```python
from build123d import *

# Parameters (mm, degrees)
F0_R     = 0.8
F1_DEPTH = 13
F2_R     = 0.8
F3_DEPTH = 6.5
F4_R     = 1.13
F5_DEPTH = 0.4


with BuildPart() as f1:
    # F0 (on Right) → F1 (new body)
    with BuildSketch(Plane.YZ):
        with BuildLine():
            ThreePointArc((0, 2.4), (-1.2, 1.2), (0, 0))
            Line((0, 0), (6.1, 0))
            Line((6.1, 0), (6.1, 0.4))
            Line((6.1, 0.4), (0.894427, 0.4))
            ThreePointArc((0.894427, 0.4), (1.095445, 1.689898), (0, 2.4))
        make_face()
        with Locations((0, 1.2)):
            Circle(F0_R, mode=Mode.SUBTRACT)
    extrude(amount=F1_DEPTH)

    # F2 (on face) → F3 (cut)
    with BuildSketch(Plane.YZ.offset(13)):
        with BuildLine():
            Line((0.894427, 0), (0.894427, 0.4))
            ThreePointArc((0.894427, 0.4), (-0.489898, 2.295445), (0, 0))
            Line((0, 0), (0.894427, 0))
        make_face()
        with Locations((0, 1.2)):
            Circle(F2_R, mode=Mode.SUBTRACT)
    extrude(amount=-F3_DEPTH, mode=Mode.SUBTRACT)

    # F4 (on face) → F5 (cut, through all)
    with BuildSketch(Plane.XY.offset(0.4)):
        with Locations((2.375, 3.67)):
            Circle(F4_R)
        with Locations((10.625, 3.67)):
            Circle(F4_R)
    extrude(amount=-F5_DEPTH, mode=Mode.SUBTRACT)


solid = f1.part
```
Geometry: final body of the model. Coordinates: model frame, mm. A direction names the side the tool comes from. Coordinates: 2 decimals unless noted, no trailing zeros. Write each loop counter-clockwise with the first axis right and the second up, starting at its lowest first coordinate (ties: lowest second). Pieces come first, ordered by that corner, then holes. Notation, with made-up numbers: M -34.5,25.25 L 1.5,25.25 A13 ccw 1.5,29.25 Z; hole C -27.5,25 d11. An arc over 180 degrees is marked long. Use CSV: the item, a comma, the result in double quotes. Start each with the question number.
1. Reachability of faces 1 (the face through (6, 3, 0)), 2 (the face through (6.5, 1, 1)) from +Z, -Z, +X, -X, +Y, -Y: full face, straight path, thin tool, end or side. Return the list, or none.
2. Ray query, probe 1 along Z at (x, y) = (2, 0); probe 2 along X at (y, z) = (3.5, 0.3); probe 3 along Z at (x, y) = (8.75, 3.5). Return the intervals inside material, ascending.
3. Cut plane C-C on x = 4.5. Return the cut outline in (y, z).
4. Cut plane B-B on y = 3.67. Return the cut outline in (x, z) (3 decimals).
5. Cut plane A-A on z = 1.2. Return the cut outline in (x, y).
6. Mould query, pull axis X, two halves, no side actions, for faces 3 (the face through (0, 1, 1)), 4 (the face through (11.15, 2.67, 0.2)), 5 (the face through (3.2, -0.17, 0.42)). Classes: pulls with the +X half, pulls with the -X half, needs draft (parallel to the pull), parting line crosses it, or undercut.
7. First-contact query: P1, Ø2.5, axis at x = 10.625, y = 3.67, coming from the +Z side; P2, Ø0.7, axis at y = 0, z = 1, coming from the +X side. Flat tips, straight axial feed; report the tip coordinate or a pass-through.
8. Cut plane D-D on y = 0.5. Return the cut outline in (x, z).
Entries:
1,face 1,"-Z, +X, -X, +Y, -Y"
1,face 2,"+Z, +X, -Y"
2,probe 1,"0 to 0.4, 2 to 2.4"
2,probe 2,"0 to 1.26, 3.49 to 9.51, 11.74 to 13"
2,probe 3,"0 to 0.4"
3,outline,"M 0,0 L 6.1,0 L 6.1,0.4 L 0.89,0.4 A1.2 ccw long Z; hole C 0,1.2 d1.6"
4,outline,"M 0,0 L 1.245,0 L 1.245,0.4 L 0,0.4 Z; M 3.505,0 L 9.495,0 L 9.495,0.4 L 3.505,0.4 Z; M 11.755,0 L 13,0 L 13,0.4 L 11.755,0.4 Z"
5,outline,"M 0,-1.2 L 6.5,-1.2 L 6.5,-0.8 L 0,-0.8 Z; M 0,0.8 L 6.5,0.8 L 6.5,1.2 L 0,1.2 Z"
6,face 3,"pulls with the -X half"
6,face 4,"undercut"
6,face 5,"needs draft"
7,P1,"z = 0.4"
7,P2,"through"
8,outline,"M 0,0 L 6.5,0 L 6.5,0.58 L 0,0.58 Z; M 0,1.82 L 6.5,1.82 L 6.5,2.29 L 0,2.29 Z"
